Can you work these out from the model? Positions are in its coordinate system, mm. Give positions to 0.01 mm unless a question says otherwise; leave off trailing zeros. Order: outer loops, then holes, each group sorted by start corner. A loop starts at its lowest first (then second) coordinate and runs counter-clockwise, first axis right, second up.
Item 1: I want a section at A-A, the plane x = -189.5. Write out the boundary of the cut face in (y, z) (1 decimal), then the cut area to 3 significant figures.
Item 2: I'm going to push flat-ended pins straight in: pin 1 Ø0.7 at (x, y) = (214, 3) entering from +Z (3 decimals); pin 2 Ø1.5 at (x, y) = (-83.5, 2.5) entering from -Z (3 decimals); pin 3 Ø1.4 at (x, y) = (-72, 1.5) entering from -Z. Where does each tip first touch, or does it pass through?
Item 3: If I drill on line 1 along X through (y, z) = (3.15, 20.5); line 2 along X through (y, z) = (3.75, 22.5); line 3 along X through (y, z) = (2.45, 13.5), over which ranges is the centre line in solid material (lowest first)?
```python
from build123d import *

# Parameters (mm, degrees)
SKETCH1_W           = 457.2
SKETCH1_H           = 47.625
BOSS_EXTRUDE1_DEPTH = 4.7625
SKETCH2_W           = 65.616666667
SKETCH2_H           = 1.5875
SKETCH2_W_2         = 105.833333333
CUT_EXTRUDE1_DEPTH  = 4.7625
SKETCH3_W           = 65.616666667
SKETCH3_H           = 1.5875
SKETCH3_W_2         = 105.833333333
CUT_EXTRUDE3_DEPTH  = 4.7625
CUT_EXTRUDE4_DEPTH  = 4.7625
SKETCH6_W           = 3.81
SKETCH6_H           = 44.45
CUT_EXTRUDE6_DEPTH  = 4.7625


with BuildPart() as part:
    # Sketch1 → Boss-Extrude1 (new body)
    with BuildSketch(Plane(origin=(0, 0, 0), x_dir=(1, 0, 0), z_dir=(0, 1, 0))):
        Rectangle(SKETCH1_W, SKETCH1_H)
    extrude(amount=BOSS_EXTRUDE1_DEPTH)

    # Sketch2 → Cut-Extrude1 (cut)
    with BuildSketch(Plane.XZ):
        with Locations((-195.791666667, 23.01875)):
            Rectangle(SKETCH2_W, SKETCH2_H)
        with Locations((-71.966666667, 23.01875)):
            Rectangle(SKETCH2_W_2, SKETCH2_H)
        with Locations((71.966666667, 23.01875)):
            Rectangle(SKETCH2_W_2, SKETCH2_H)
        with Locations((195.791666667, 23.01875)):
            Rectangle(SKETCH2_W, SKETCH2_H)
    extrude(amount=-CUT_EXTRUDE1_DEPTH, mode=Mode.SUBTRACT)

    # Sketch3 → Cut-Extrude3 (cut)
    with BuildSketch(Plane.XZ):
        with Locations((-195.791666667, -23.01875)):
            Rectangle(SKETCH3_W, SKETCH3_H)
        with Locations((-71.966666667, -23.01875)):
            Rectangle(SKETCH3_W_2, SKETCH3_H)
        with Locations((71.966666667, -23.01875)):
            Rectangle(SKETCH3_W_2, SKETCH3_H)
        with Locations((195.791666667, -23.01875)):
            Rectangle(SKETCH3_W, SKETCH3_H)
    extrude(amount=-CUT_EXTRUDE3_DEPTH, mode=Mode.SUBTRACT)

    # Sketch4 → Cut-Extrude4 (cut)
    with BuildSketch(Plane(origin=(0, 4.7625, 0), x_dir=(1, 0, 0), z_dir=(0, 1, 0))):
        Polygon((217.32875, -22.225), (214.47125, -22.225), (214.47125, -14.605), (213.106, -14.605), (213.106, -10.795), (214.47125, -10.795), (214.47125, -3.683), (217.32875, -3.683), (217.32875, -10.795), (218.694, -10.795), (218.694, -14.605), (217.32875, -14.605), align=None)
        Polygon((73.395413242, -22.225), (73.395413242, -15.940182767), (74.760663242, -15.940182767), (74.760663242, -12.094601121), (73.395413242, -12.094601121), (73.395413242, -3.677534747), (70.537920091, -3.677534747), (70.537920091, -12.094601121), (69.172670091, -12.094601121), (69.172670091, -15.940182767), (70.537920091, -15.940182767), (70.537920091, -22.225), align=None)
        Polygon((-70.537916667, -22.225), (-70.537916667, -14.605), (-69.172666667, -14.605), (-69.172666667, -10.795), (-70.537916667, -10.795), (-70.537916667, -3.683), (-73.395416667, -3.683), (-73.395416667, -10.795), (-74.760666667, -10.795), (-74.760666667, -14.605), (-73.395416667, -14.605), (-73.395416667, -22.225), align=None)
        Polygon((-214.47125, -22.225), (-214.47125, -14.605), (-213.106, -14.605), (-213.106, -10.795), (-214.47125, -10.795), (-214.47125, -3.683), (-217.32875, -3.683), (-217.32875, -10.795), (-218.694, -10.795), (-218.694, -14.605), (-217.32875, -14.605), (-217.32875, -22.225), align=None)
        Polygon((-214.47125, 22.225), (-217.32875, 22.225), (-217.32875, 14.605), (-218.694, 14.605), (-218.694, 10.795), (-217.32875, 10.795), (-217.32875, 3.683), (-214.47125, 3.683), (-214.47125, 10.795), (-213.106, 10.795), (-213.106, 14.605), (-214.47125, 14.605), align=None)
        Polygon((-69.172666667, 14.605), (-70.537916667, 14.605), (-70.537916667, 22.225), (-73.395416667, 22.225), (-73.395416667, 14.605), (-74.760666667, 14.605), (-74.760666667, 10.795), (-73.395416667, 10.795), (-73.395416667, 3.683), (-70.537916667, 3.683), (-70.537916667, 10.795), (-69.172666667, 10.795), align=None)
        Polygon((74.760663242, 15.940182767), (73.395413242, 15.940182767), (73.395413242, 22.225), (70.537920091, 22.225), (70.537920091, 15.940182767), (69.172670091, 15.940182767), (69.172670091, 12.094601121), (70.537920091, 12.094601121), (70.537920091, 3.677534747), (73.395413242, 3.677534747), (73.395413242, 12.094601121), (74.760663242, 12.094601121), align=None)
        Polygon((218.694, 10.795), (217.32875, 10.795), (217.32875, 3.683), (214.47125, 3.683), (214.47125, 10.795), (213.106, 10.795), (213.106, 14.605), (214.47125, 14.605), (214.47125, 22.225), (217.32875, 22.225), (217.32875, 14.605), (218.694, 14.605), align=None)
    extrude(amount=-CUT_EXTRUDE4_DEPTH, mode=Mode.SUBTRACT)

    # Sketch6 → Cut-Extrude6 (cut)
    with BuildSketch(Plane(origin=(0, 4.7625, 0), x_dir=(1, 0, 0), z_dir=(0, 1, 0))):
        with Locations((-226.695, 0)):
            Rectangle(SKETCH6_W, SKETCH6_H)
        with Locations((226.695, 0)):
            Rectangle(SKETCH6_W, SKETCH6_H)
    extrude(amount=-CUT_EXTRUDE6_DEPTH, mode=Mode.SUBTRACT)


solid = part.part
```
Results list:
1. outline: (0, -22.2) - (4.8, -22.2) - (4.8, 22.2) - (0, 22.2) - close
1. area: 212 mm2
2. pin 1: stops at z = 22.225
2. pin 2: stops at z = -22.225
2. pin 3: stops at z = -3.68
3. line 1: x = -224.79 to -217.33, -214.47 to -73.4, -70.54 to 70.54, 73.4 to 214.47, 217.33 to 224.79
3. line 2: x = -162.98 to -124.88, -19.05 to 19.05, 124.88 to 162.98
3. line 3: x = -224.79 to -218.69, -213.11 to -74.76, -69.17 to 69.17, 74.76 to 213.11, 218.69 to 224.79
